Part print with two shaded views. Sizes in mm from the minimum x, y, z corner. A direction names the side the tool comes from. Coordinates: 2 decimals unless noted, no trailing zeros. Loops run counter-clockwise (first coordinate to the right, second up) from the corner with the lowest first, then second, coordinate; pieces in that order, holes last.
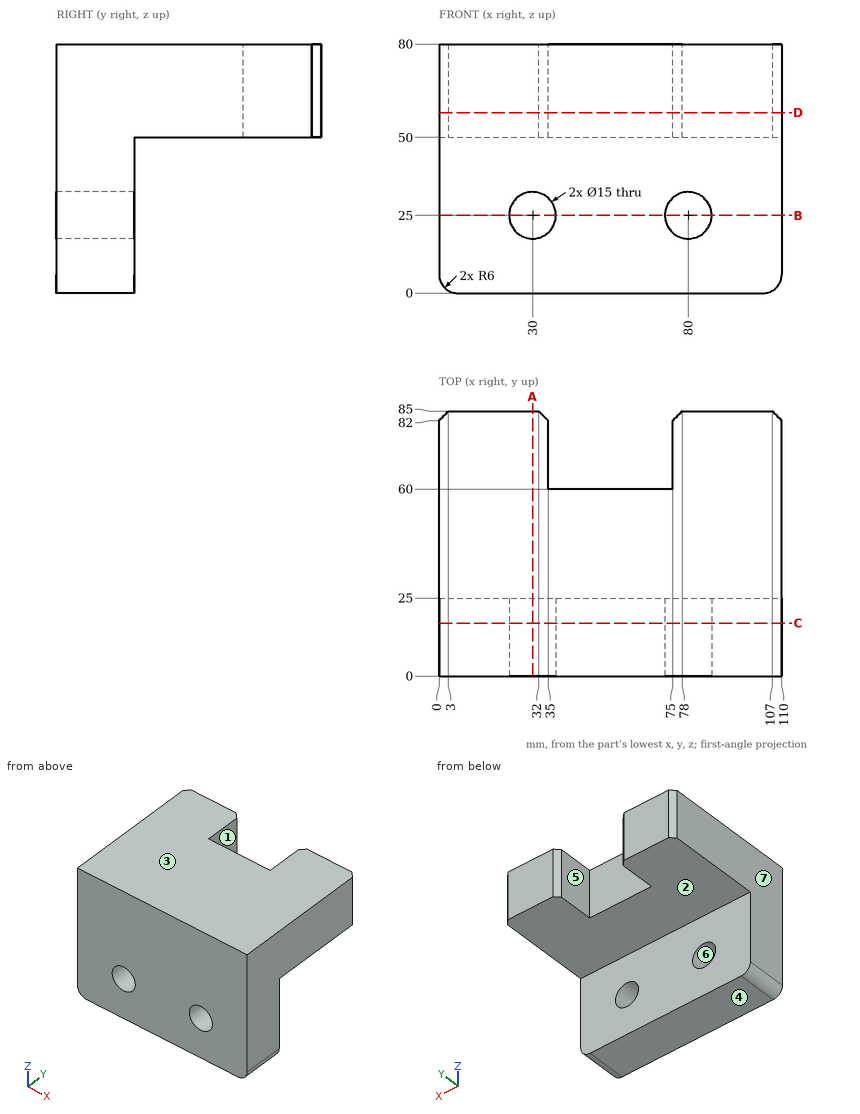
Q1. Slice it at D-D (z = 58). List the corners of the cut face in (x, y).
Answers:
outline: (0, 0) - (110, 0) - (110, 82) - (107, 85) - (78, 85) - (75, 82) - (75, 60) - (35, 60) - (35, 82) - (32, 85) - (3, 85) - (0, 82) - close
Q2. Flat gauge pins, fed straight in: P1, Ø13.5, axis at x = 30, z = 25, coming from the -Y side; P2, Ø3, axis at x = 41.5, z = 53.5, coming from the +Y side; P3, Ø10, axis at x = 85.5, y = 68, coming from the -Z side; P4, Ø10, axis at x = 18.5, z = 9, coming from the +Y side. Where does each tip first touch, or does it go through?
Answers:
P1: passes through
P2: stops at y = 60
P3: stops at z = 50
P4: stops at y = 25
Q3. Drill centre lines: line 1 (X direction, y = 17.5, z = 25); line 2 (Z direction, x = 80, y = 5.75); line 3 (X direction, y = 10, z = 20). Where is each one in solid material? Low to high.
Answers:
line 1: x = 0 to 22.5, 37.5 to 72.5, 87.5 to 110
line 2: z = 0 to 17.5, 32.5 to 80
line 3: x = 0 to 24.41, 35.59 to 74.41, 85.59 to 110
Q4. Slice it at A-A (x = 30). List the corners of the cut face in (y, z).
Answers:
outline: (0, 0) - (25, 0) - (25, 17.5) - (0, 17.5) - close; (0, 32.5) - (25, 32.5) - (25, 50) - (85, 50) - (85, 80) - (0, 80) - close
Q5. Slice it at C-C (y = 17). List the corners of the cut face in (x, z).
Answers:
outline: (0, 6) arc R6 ccw to (6, 0) - (104, 0) arc R6 ccw to (110, 6) - (110, 80) - (0, 80) - close; hole circle Ø15 at (30, 25); hole circle Ø15 at (80, 25)
Q6. Slice it at B-B (z = 25). List the corners of the cut face in (x, y), and give its area (3 significant figures).
Answers:
outline: (0, 0) - (22.5, 0) - (22.5, 25) - (0, 25) - close; (37.5, 0) - (72.5, 0) - (72.5, 25) - (37.5, 25) - close; (87.5, 0) - (110, 0) - (110, 25) - (87.5, 25) - close
area: 2,000 mm2
Q7. Which spindle directions (+Z, -Z, +X, -X, +Y, -Y) get a long thin tool onto all of the face, cutting with end or side? Do the marked faces 1, 2 and 3. Say none if no direction does.
Answers:
face 1: +Z, -Z, +Y
face 2: -Z, +X, -X, +Y
face 3: +Z, +X, -X, +Y, -Y
Q8. Mould opens along X. For the marked faces 4, 5, 6 and 7 say: +X half, -X half, draft (parallel to the pull), parting line (faces both ways), or undercut.
Answers:
face 4: draft
face 5: undercut
face 6: undercut
face 7: -X half
